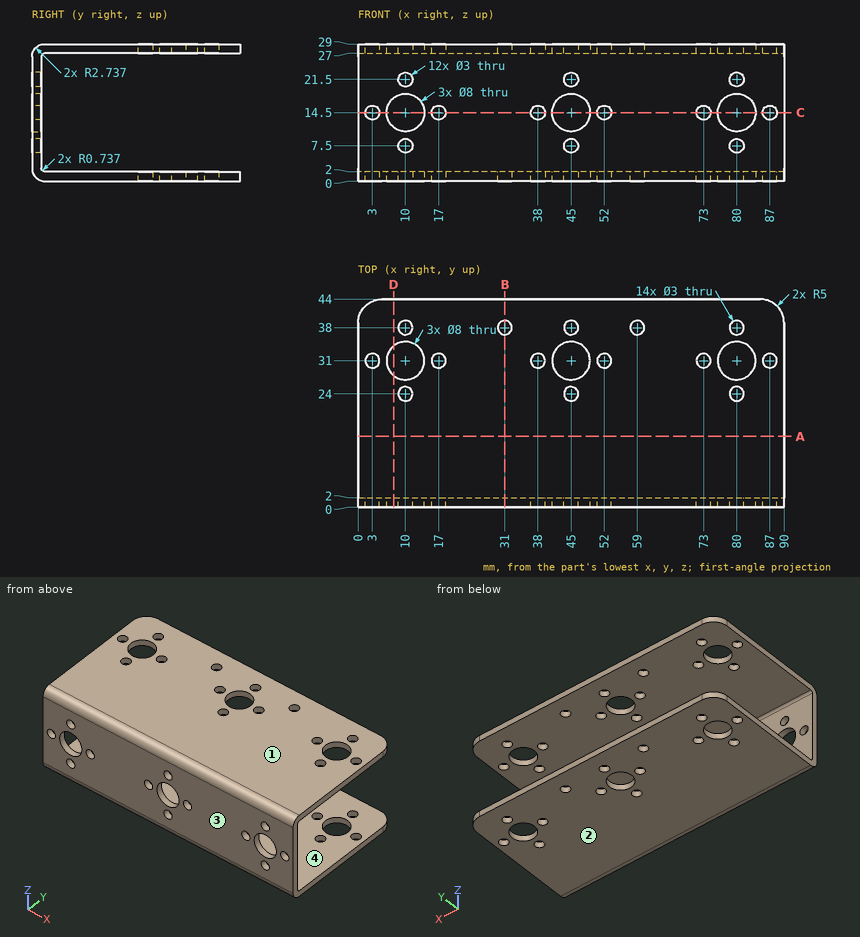
Geometry: see drawing. Coordinates: mm, zero at the bounding-box minimum. Coordinates: 2 decimals unless noted, no trailing zeros. Loops run counter-clockwise (first coordinate to the right, second up) from the corner with the lowest first, then second, coordinate; pieces in that order, holes last.
Q1. Cut plane B-B (x = 31). Output: boundary loops of the cut face in (y, z), then the cut area to 3 significant figures.
Q2. Cut plane D-D (x = 7.5). Output: boundary loops of the cut face in (y, z).
Q3. Cut plane C-C (z = 14.5). Give the number of separate pieces and of enclosed holes in the cut face.
Q4. Contact query for flat-ended pins moving along their axis: pin 1 (2.5 mm diameter, centred on x = 45, y = 24, fed in from -Z); pin 2 (1.5 mm diameter, centred on x = 66, z = 9, fed in from +Y); pin 3 (12 mm diameter, centred on x = 33.5, z = 21.5, fed in from +Y). Output: stop coordinate, or through.
Q5. Material intervals for line 1 (Z direction, x = 49, y = 18.5); line 2 (Y direction, x = 80, z = 0.9); line 3 (Y direction, x = 30, z = 25.75), sorted ascending.
Q6. Cut plane A-A (y = 15). Output: boundary loops of the cut face in (x, z).
Q7. Draft query along Z for the marked faces 1, 2, 3 and 4. Return one class per face: +Z half, -Z half, draft (parallel to the pull), parting line (faces both ways), or undercut.
Working result:
1. outline: (0, 2.74) arc R2.74 ccw to (2.74, 0) - (36.5, 0) - (36.5, 2) - (2.74, 2) arc R0.74 cw to (2, 2.74) - (2, 26.26) arc R0.74 cw to (2.74, 27) - (36.5, 27) - (36.5, 29) - (2.74, 29) arc R2.74 ccw to (0, 26.26) - close; (39.5, 0) - (44, 0) - (44, 2) - (39.5, 2) - close; (39.5, 27) - (44, 27) - (44, 29) - (39.5, 29) - close
1. area: 211 mm2
2. outline: (0, 2.74) arc R2.74 ccw to (2.74, 0) - (27.88, 0) - (27.88, 2) - (2.74, 2) arc R0.74 cw to (2, 2.74) - (2, 11.38) - (0, 11.38) - close; (0, 17.62) - (2, 17.62) - (2, 26.26) arc R0.74 cw to (2.74, 27) - (27.88, 27) - (27.88, 29) - (2.74, 29) arc R2.74 ccw to (0, 26.26) - close; (34.12, 0) - (44, 0) - (44, 2) - (34.12, 2) - close; (34.12, 27) - (44, 27) - (44, 29) - (34.12, 29) - close
3. separate pieces: 10
3. enclosed holes: 0
4. pin 1: passes through
4. pin 2: stops at y = 2
4. pin 3: stops at y = 44
5. line 1: z = 0 to 2, 27 to 29
5. line 2: y = 0.71 to 22.5, 25.5 to 27, 35 to 36.5, 39.5 to 44
5. line 3: y = 0 to 2
6. outline: (0, 0) - (90, 0) - (90, 2) - (0, 2) - close; (0, 27) - (90, 27) - (90, 29) - (0, 29) - close
7. face 1: +Z half
7. face 2: -Z half
7. face 3: draft
7. face 4: undercut
